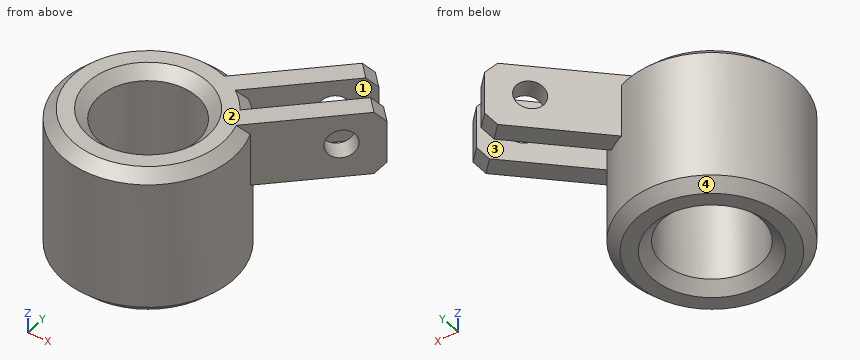
Autodesk Inventor part; units mm, degrees
ref_plane "YZ Plane" through (0, 0, 0) normal (1, 0, 0) x (0, 1, 0)
ref_plane "XZ Plane" through (0, 0, 0) normal (0, 1, 0) x (-1, 0, 0)
ref_plane "XY Plane" through (0, 0, 0) normal (0, 0, 1) x (1, 0, 0)
sketch "Эскиз1" plane through (0, 0, 0) normal (0, 0, 1) x (1, 0, 0)
  circle A0 centre (0, 0) radius 8.1
  circle A1 centre (0, 0) radius 8
  circle A2 centre (0, 0) radius 4.6
  dimension "d0" = 0.1
  dimension "d1" = 9.2
extrude "Выдавливание1" add sketch "Эскиз1" along normal blind 14 contours A1
chamfer "Фаска1" distance 1 angle 45 4 edges at (-8, 0, 14) (-8, 0, 0) (-4.6, 0, 14) (-4.6, 0, 0)
sketch "Эскиз2" plane through (0, 0, 14) normal (0, 0, 1) x (1, 0, 0)
  circle A0 centre (15.2735, -186.1533) radius 2.5
  circle A1 centre (19.2813, -181.6882) radius 2.5
  circle A2 centre (6.7164, -177.6929) radius 2.5
  circle A3 centre (6.7164, -107.6929) radius 2.5
  circle A4 centre (11.2658, -120.6185) radius 2.5
  circle A5 centre (6.7164, -37.6929) radius 2.5
  circle A6 centre (15.2735, -46.1533) radius 2.5
  circle A7 centre (23.2891, -37.223) radius 2.5
  circle A8 centre (26, -154.7115) radius 6
  circle A9 centre (26, -84.7115) radius 6
  circle A10 centre (-32.5, -91.359) radius 1.5
  circle A11 centre (-32.5, -21.359) radius 1.5
  line L0 (15.5395, 14.1253) -> (7.4584, 6.0442)
  arc A12 (6.0442, 7.4584) -> (7.4584, 6.0442) centre (0, 0) ccw
  line L1 (6.0442, 7.4584) -> (14.1253, 15.5395)
  arc A13 (14.1253, 15.5395) -> (-20.9712, 1.0986) centre (0, 0) ccw
  arc A14 (-25.0526, -8.0684) -> (-20.9712, 1.0986) centre (-34.9521, 1.8311) ccw
  line L2 (-25.0526, -8.0684) -> (-27.881, -10.8968)
  line L3 (-27.881, -5.24) -> (-27.881, -10.8968)
  line L4 (-36.4645, -13.8234) -> (-27.881, -5.24)
  line L5 (-39, -19.9448) -> (-36.4645, -13.8234)
  line L6 (-39, -107.9932) -> (-39, -19.9448)
  line L7 (-38.7059, -110.2271) -> (-39, -107.9932)
  line L8 (-11.2941, -212.5294) -> (-38.7059, -110.2271)
  line L9 (-10, -222.359) -> (-11.2941, -212.5294)
  line L10 (-10, -239.5306) -> (-10, -222.359)
  line L11 (-5.9, -243.6306) -> (-10, -239.5306)
  line L12 (-5.9, -232.3168) -> (-5.9, -243.6306)
  line L13 (-5.9, -232.3168) -> (-1.4533, -236.7636)
  arc A15 (-0.3274, -237.8894) -> (-1.4533, -236.7636) centre (0.6355, -235.8007) ccw
  line L14 (-0.3274, -237.8894) -> (0.1419, -238.3587)
  line L15 (0.1419, -238.3587) -> (21.8181, -232.5506)
  arc A16 (21.8181, -232.5506) -> (28.9814, -229.4318) centre (15, -207.1051) ccw
  arc A17 (32.6098, -226.6973) -> (28.9814, -229.4318) centre (30.5792, -227.7773) ccw
  arc A18 (32.6098, -226.6973) -> (41.3431, -207.1051) centre (15, -207.1051) ccw
  line L16 (41.3431, -207.1051) -> (41.3431, -44.3275)
  line L17 (40.8708, -43.2834) -> (41.3431, -44.3275)
  line L18 (40.8708, -43.2834) -> (30.4465, -37.265)
  spline S0 degree 3 poles (30.4465, -37.265) (28.5259, -36.1561) (26.8693, -34.6988) (23.9575, -31.0426) (22.8201, -28.8572) (21.6341, -25.5426) (21.3338, -24.5174) (21.0841, -23.4772) knots -1.71756 -1.71756 -1.71756 -1.71756 -1.05224 -1.05224 -0.317791 -0.317791 0 0 0 0
  arc A19 (20.3792, -6.3803) -> (21.0841, -23.4772) centre (26, -14.7115) ccw
  spline S1 degree 3 poles (20.3792, -6.3803) (20.4968, -5.2098) (20.6383, -4.0488) (20.7981, -2.9054) knots -3.756173 -3.756173 -3.756173 -3.756173 -3.409835 -3.409835 -3.409835 -3.409835
  arc A20 (20.7981, -2.9054) -> (15.5395, 14.1253) centre (0, 0) ccw
  circle A21 centre (19.2813, -41.6882) radius 2.5
  circle A22 centre (11.2658, -50.6185) radius 2.5
  circle A23 centre (19.2813, -111.6882) radius 2.5
  circle A24 centre (15.2735, -116.1533) radius 2.5
  circle A25 centre (23.2891, -107.223) radius 2.5
  circle A26 centre (23.2891, -177.223) radius 2.5
  circle A27 centre (11.2658, -190.6185) radius 2.5
  circle A28 centre (11.5956, -216.8171) radius 12.85
  circle A29 centre (-7.3879, -205.857) radius 2.3
  circle A30 centre (22.5558, -197.8336) radius 2.3
  circle A31 centre (0, 0) radius 8
  line L19 (2.3508, 6.5935) -> (12.5756, 16.8183)
  line L20 (6.0442, 7.4584) -> (4.1919, 5.6061)
  line L21 (11.9803, 13.3945) -> (10.5661, 14.8088)
  line L22 (10.5661, 11.9803) -> (11.9803, 10.5661)
  circle A32 centre (0, 0) radius 7
  line L23 (0, 0) -> (10.0847, 10.0847)
  line L24 (6.5935, 2.3508) -> (16.8183, 12.5756)
  line L25 (7.4584, 6.0442) -> (5.6061, 4.1919)
  line L26 (13.3945, 11.9803) -> (14.8088, 10.5661)
  line L27 (4.0279, 5.725) -> (11.8389, 13.536)
  line L28 (5.725, 4.0279) -> (13.536, 11.8389)
  point P0 (6.5935, 2.3508)
  dimension "d7" = 2
  dimension "d8" = 2
  dimension "d14" = 0.2
  dimension "d15" = 0.2
extrude "Выдавливание2" add sketch "Эскиз2" against normal blind 6 contours L26 L24 A12 L28 | A12 L24 A31 L28 | A31 L24 A32 L28 | L19 L21 L27 A12 | A12 L27 A31 L19 | A31 L27 A32 L19
chamfer "Фаска2" distance 1 angle 45 4 edges at (11.2025, 14.1724, 14) (11.2025, 14.1724, 8) (14.1724, 11.2025, 14) (14.1724, 11.2025, 8)
sketch "Эскиз3" plane through (3.1227, 7.3654, 8) normal (-0.7071, 0.7071, 0) x (-0.7071, -0.7071, 0)
  circle A0 centre (-7.0266, 3.2) radius 1.5
  circle A1 centre (-7.0266, 3.2) radius 1.35
  point P0 (7.4162, -8)
  dimension "d18" = 2.7
extrude "Выдавливание3" cut sketch "Эскиз3" against normal blind 6 contours A1
properties part number "Втулка"
Check sheet for the modelled part. Datum: model origin and axes. Units: mm. Face numbers are marked on the shaded views. Give positions to 0.01 mm unless a question says otherwise; leave off trailing zeros. Order: outer loops, then holes, each group sorted by start corner. A loop starts at its lowest first (then second) coordinate and runs counter-clockwise, first axis right, second up. Notation, with made-up numbers: M 50.5,-27.75 L 76.5,-27.75 A26 ccw 76.5,2.25 Z; hole C 79,-16 d1. An arc over 180 degrees is marked long. Answer in a Markdown table with one row per item.
1) Cross-section at D-D, the plane z = 12. Enter the section's corners in (x, y), plus the area to 3 significant figures.
Filled sheet:
| item | result |
|---|---|
| outline | M 3.12,7.37 A8 ccw long 7.37,3.12 L 11.57,7.32 L 10.29,8.6 L 6.44,4.74 A8 ccw 4.74,6.44 L 8.6,10.29 L 7.32,11.57 Z; M 8.86,13.1 L 10.13,11.83 L 11.84,13.54 L 10.57,14.81 Z; M 11.83,10.13 L 13.1,8.86 L 14.81,10.57 L 13.54,11.84 Z; hole C 0,0 d9.2 |
| area | 164 mm2 |
2) Gauge pin test, flat ends, axial feed: P1, Ø1.5, axis at x = -1, z = 4.5, coming from the -Y side; P2, Ø5, axis at y = 4.5, z = 7, coming from the +X side; P3, Ø3, axis at y = 8.5, z = 1.5, coming from the +X side. Record the tip position at first contact, or that the pin passes through.
Filled sheet:
| item | result |
|---|---|
| P1 | stops at y = -8 |
| P2 | stops at x = 11.03 |
| P3 | stops at x = 3.87 |
3) Cross-section at C-C, the plane z = 4.75. Enter the section's corners in (x, y).
Filled sheet:
| item | result |
|---|---|
| outline | C 0,0 d16; hole C 0,0 d9.2 |
4) Cross-section at A-A, the plane z = 10.5. Enter the section's corners in (x, y).
Filled sheet:
| item | result |
|---|---|
| outline | M 3.12,7.37 A8 ccw long 7.37,3.12 L 11.52,7.28 L 10.24,8.55 L 6.44,4.74 A8 ccw 4.74,6.44 L 8.55,10.24 L 7.28,11.52 Z; M 8.91,13.15 L 10.18,11.88 L 11.84,13.54 L 10.57,14.81 Z; M 11.88,10.18 L 13.15,8.91 L 14.81,10.57 L 13.54,11.84 Z; hole C 0,0 d9.2 |
5) Thickness scan on L1, parallel to Y at x = 0, z = 7; L2, parallel to X at y = 0.25, z = 3.5; L3, parallel to Y at x = -2.25, z = 12.5. Record the ranges inside material, lowest first. Write a range as [from, to].
Filled sheet:
| item | result |
|---|---|
| L1 | y = [-8, -4.6], [4.6, 8] |
| L2 | x = [-8, -4.59], [4.59, 8] |
| L3 | y = [-7.68, -4.01], [4.01, 7.68] |
6) Cross-section at B-B, the plane x = 0. Enter the section's corners in (y, z).
Filled sheet:
| item | result |
|---|---|
| outline | M -8,1 L -7,0 L -5.6,0 L -4.6,1 L -4.6,13 L -5.6,14 L -7,14 L -8,13 Z; M 4.6,1 L 5.6,0 L 7,0 L 8,1 L 8,13 L 7,14 L 5.6,14 L 4.6,13 Z |
7) Release check for a two-part mould opening along Y. For the marked faces 1, 2, 3 and 4 record: +Y half, -Y half, draft (parallel to the pull), parting line (faces both ways), or undercut.
Filled sheet:
| item | result |
|---|---|
| face 1 | undercut |
| face 2 | draft |
| face 3 | undercut |
| face 4 | parting line |
